Verification items for this drawing (mm, ordinates from the low corner). Coordinates: 2 decimals unless noted, no trailing zeros. Write each loop counter-clockwise with the first axis right and the second up, starting at its lowest first coordinate (ties: lowest second). Pieces come first, ordered by that corner, then holes. Notation, with made-up numbers: (83, 49.5) -> (127, 49.5) arc R19 cw to (127, 67.5) -> close; hole circle Ø10 at (-27.5, 88). An arc over 180 degrees is marked (long way). One line per question, with ' | ' between items.
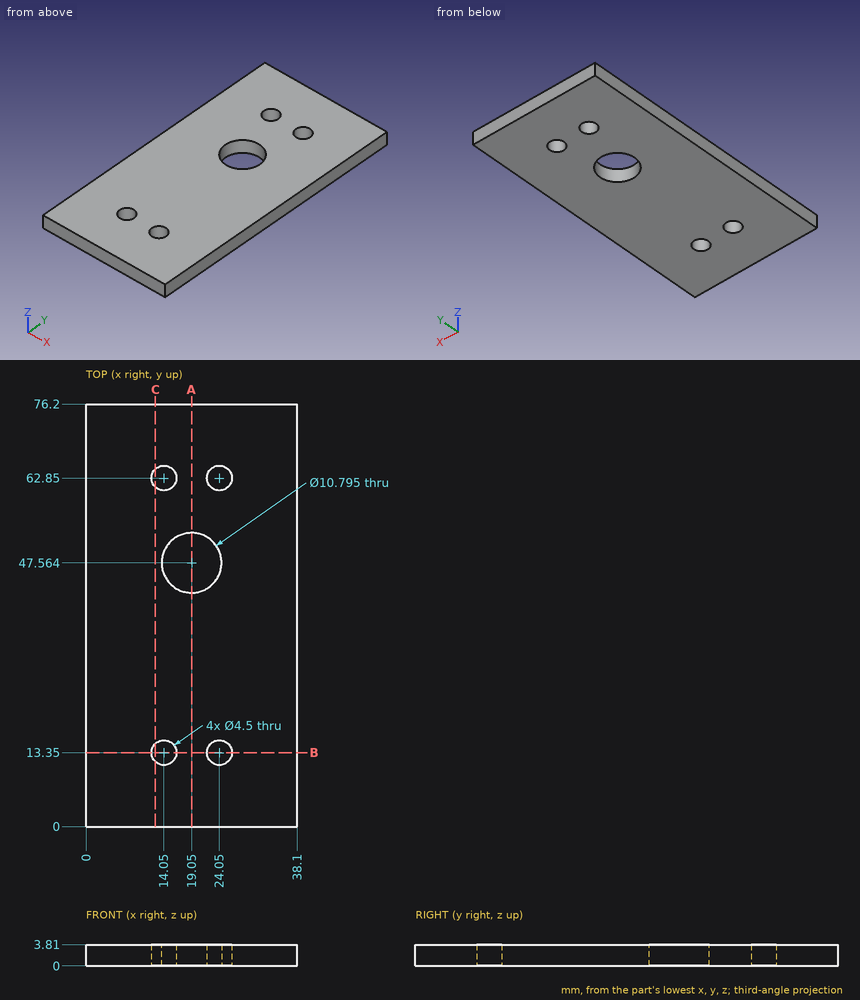
(1) Cross-section at C-C (x = 12.5). Record the cut outline in (y, z).
Answers below:
outline: (0, 0) -> (11.72, 0) -> (11.72, 3.81) -> (0, 3.81) -> close; (14.98, 0) -> (61.22, 0) -> (61.22, 3.81) -> (14.98, 3.81) -> close; (64.48, 0) -> (76.2, 0) -> (76.2, 3.81) -> (64.48, 3.81) -> close
(2) Cross-section at A-A (x = 19.05). Record the cut outline in (y, z).
Answers below:
outline: (0, 0) -> (42.17, 0) -> (42.17, 3.81) -> (0, 3.81) -> close; (52.96, 0) -> (76.2, 0) -> (76.2, 3.81) -> (52.96, 3.81) -> close
(3) Cross-section at B-B (y = 13.35). Record the cut outline in (x, z), plus the area to 3 significant figures.
Answers below:
outline: (0, 0) -> (11.8, 0) -> (11.8, 3.81) -> (0, 3.81) -> close; (16.3, 0) -> (21.8, 0) -> (21.8, 3.81) -> (16.3, 3.81) -> close; (26.3, 0) -> (38.1, 0) -> (38.1, 3.81) -> (26.3, 3.81) -> close | area: 111 mm²
(4) Material ranges on line 1 (Y direction, x = 19.05, z = 1.6); line 2 (Y direction, x = 24.5, z = 0.95); line 3 (Y direction, x = 23.5, z = 2.2), recorded low to high.
Answers below:
line 1: y = 0 to 42.17, 52.96 to 76.2 | line 2: y = 0 to 11.15, 15.55 to 60.65, 65.05 to 76.2 | line 3: y = 0 to 11.17, 15.53 to 44.51, 50.62 to 60.67, 65.03 to 76.2
